Build history of the part. All positions in model axes, mm. Coordinates: 2 decimals unless noted, no trailing zeros. Loops run counter-clockwise (first coordinate to the right, second up) from the corner with the lowest first, then second, coordinate; pieces in that order, holes last.
Item 1: Cut at A-A (x = 63.5). List the corners of the cut face in (y, z) (3 decimals), and give its area (3 significant figures).
Item 2: Mould opens along X. For faces 1 (the face through (48, 12.7, -64)), 2 (the face through (67.315, 14.31, -51.386)), 3 (the face through (45.73, 6.44, -56.52)) say: released by +X, released by -X, zero draft, split by the parting line, or undercut.
Item 3: Cut at C-C (x = 30.5). List the corners of the cut face in (y, z).
Item 4: Drill centre lines: line 1 along Y through (x, z) = (41.5, -44.5); line 2 along X through (y, z) = (10, -51); line 3 along Z through (x, y) = (51.5, 7). Where is each one in solid material? Low to high.
Item 5: Cut at D-D (z = -96.5). List the corners of the cut face in (x, y), and give its area (3 significant figures).
Item 6: Flat gauge pins, fed straight in: pin 1 (3 mm diameter, centred on x = 68.73, z = -45.18, fed in from +Y); pin 2 (4 mm diameter, centred on x = 58.27, z = -45.18, fed in from +Y). Where does each tip first touch, or does it go through?
Item 7: Cut at B-B (z = -63.5). List the corners of the cut face in (x, y) (3 decimals).
from build123d import *

# Parameters (mm, degrees)
SKETCH3_W           = 127
SKETCH3_H           = 127
BOSS_EXTRUDE1_DEPTH = 15.875
SKETCH4_W           = 127
SKETCH4_H           = 127
SKETCH4_R           = 12.7
CUT_EXTRUDE1_DEPTH  = 3.175
CUT_EXTRUDE2_REACH  = 182.054
SKETCH5_R           = 1.8288
CUT_EXTRUDE3_REACH  = 182.054
SKETCH9_R           = 1.8288
CUT_EXTRUDE4_REACH  = 182.054
SKETCH10_R          = 1.8288


with BuildPart() as part:
    # Sketch3 → Boss-Extrude1 (new body)
    with BuildSketch(Plane(origin=(0, 0, 0), x_dir=(1, 0, 0), z_dir=(0, 1, 0))):
        with Locations((63.5, 63.5)):
            Rectangle(SKETCH3_W, SKETCH3_H)
    extrude(amount=BOSS_EXTRUDE1_DEPTH)

    # Sketch4 → Cut-Extrude1 (cut)
    with BuildSketch(Plane(origin=(0, 15.875, 0), x_dir=(1, 0, 0), z_dir=(0, 1, 0))):
        with Locations((63.5, 63.5)):
            Rectangle(SKETCH4_W, SKETCH4_H)
        with Locations(Location((63.5, 63.5, 0), (0, 0, 270))):
            Circle(SKETCH4_R, mode=Mode.SUBTRACT)
    extrude(amount=-CUT_EXTRUDE1_DEPTH, mode=Mode.SUBTRACT)

    # Sketch5 → Cut-Extrude2 (cut, up to next)
    with BuildSketch(Plane(origin=(0, 12.7, 0), x_dir=(1, 0, 0), z_dir=(0, 1, 0)), mode=Mode.PRIVATE) as cut_extrude2_sk1:
        with Locations(Location((45.182968797, 58.266562514, 0), (0, 0, 270))):
            Circle(SKETCH5_R)
    cut_extrude2_tool1 = extrude(cut_extrude2_sk1.sketch, amount=-CUT_EXTRUDE2_REACH, mode=Mode.PRIVATE) & part.part
    # Sketch5 → Cut-Extrude2 (cut, up to next)
    with BuildSketch(Plane(origin=(0, 12.7, 0), x_dir=(1, 0, 0), z_dir=(0, 1, 0)), mode=Mode.PRIVATE) as cut_extrude2_sk2:
        with Locations(Location((68.733437486, 45.182968797, 0), (0, 0, 270))):
            Circle(SKETCH5_R)
    cut_extrude2_tool2 = extrude(cut_extrude2_sk2.sketch, amount=-CUT_EXTRUDE2_REACH, mode=Mode.PRIVATE) & part.part
    # Sketch5 → Cut-Extrude2 (cut, up to next)
    with BuildSketch(Plane(origin=(0, 12.7, 0), x_dir=(1, 0, 0), z_dir=(0, 1, 0)), mode=Mode.PRIVATE) as cut_extrude2_sk3:
        with Locations(Location((81.817031203, 68.733437486, 0), (0, 0, 270))):
            Circle(SKETCH5_R)
    cut_extrude2_tool3 = extrude(cut_extrude2_sk3.sketch, amount=-CUT_EXTRUDE2_REACH, mode=Mode.PRIVATE) & part.part
    # Sketch5 → Cut-Extrude2 (cut, up to next)
    with BuildSketch(Plane(origin=(0, 12.7, 0), x_dir=(1, 0, 0), z_dir=(0, 1, 0)), mode=Mode.PRIVATE) as cut_extrude2_sk4:
        with Locations(Location((58.266562514, 81.817031203, 0), (0, 0, 270))):
            Circle(SKETCH5_R)
    cut_extrude2_tool4 = extrude(cut_extrude2_sk4.sketch, amount=-CUT_EXTRUDE2_REACH, mode=Mode.PRIVATE) & part.part
    add(cut_extrude2_tool1.solids().sort_by_distance((45.182969, 12.7, -58.266563))[0], mode=Mode.SUBTRACT)
    add(cut_extrude2_tool2.solids().sort_by_distance((68.733437, 12.7, -45.182969))[0], mode=Mode.SUBTRACT)
    add(cut_extrude2_tool3.solids().sort_by_distance((81.817031, 12.7, -68.733437))[0], mode=Mode.SUBTRACT)
    add(cut_extrude2_tool4.solids().sort_by_distance((58.266563, 12.7, -81.817031))[0], mode=Mode.SUBTRACT)

    # Sketch9 → Cut-Extrude3 (cut, up to next)
    with BuildSketch(Plane(origin=(0, 12.7, 0), x_dir=(1, 0, 0), z_dir=(0, 1, 0)), mode=Mode.PRIVATE) as cut_extrude3_sk1:
        with Locations(Location((68.733437486, 81.817031203, 0), (0, 0, 270))):
            Circle(SKETCH9_R)
    cut_extrude3_tool1 = extrude(cut_extrude3_sk1.sketch, amount=-CUT_EXTRUDE3_REACH, mode=Mode.PRIVATE) & part.part
    # Sketch9 → Cut-Extrude3 (cut, up to next)
    with BuildSketch(Plane(origin=(0, 12.7, 0), x_dir=(1, 0, 0), z_dir=(0, 1, 0)), mode=Mode.PRIVATE) as cut_extrude3_sk2:
        with Locations(Location((58.266562514, 45.182968797, 0), (0, 0, 270))):
            Circle(SKETCH9_R)
    cut_extrude3_tool2 = extrude(cut_extrude3_sk2.sketch, amount=-CUT_EXTRUDE3_REACH, mode=Mode.PRIVATE) & part.part
    add(cut_extrude3_tool1.solids().sort_by_distance((68.733437, 12.7, -81.817031))[0], mode=Mode.SUBTRACT)
    add(cut_extrude3_tool2.solids().sort_by_distance((58.266563, 12.7, -45.182969))[0], mode=Mode.SUBTRACT)

    # Sketch10 → Cut-Extrude4 (cut, up to next)
    with BuildSketch(Plane(origin=(0, 12.7, 0), x_dir=(1, 0, 0), z_dir=(0, 1, 0)), mode=Mode.PRIVATE) as cut_extrude4_sk1:
        with Locations(Location((76.970384182, 76.970384182, 0), (0, 0, 270))):
            Circle(SKETCH10_R)
    cut_extrude4_tool1 = extrude(cut_extrude4_sk1.sketch, amount=-CUT_EXTRUDE4_REACH, mode=Mode.PRIVATE) & part.part
    # Sketch10 → Cut-Extrude4 (cut, up to next)
    with BuildSketch(Plane(origin=(0, 12.7, 0), x_dir=(1, 0, 0), z_dir=(0, 1, 0)), mode=Mode.PRIVATE) as cut_extrude4_sk2:
        with Locations(Location((50.029615818, 50.029615818, 0), (0, 0, 270))):
            Circle(SKETCH10_R)
    cut_extrude4_tool2 = extrude(cut_extrude4_sk2.sketch, amount=-CUT_EXTRUDE4_REACH, mode=Mode.PRIVATE) & part.part
    add(cut_extrude4_tool1.solids().sort_by_distance((76.970384, 12.7, -76.970384))[0], mode=Mode.SUBTRACT)
    add(cut_extrude4_tool2.solids().sort_by_distance((50.029616, 12.7, -50.029616))[0], mode=Mode.SUBTRACT)


solid = part.part
Filled sheet:
1. outline: (0, -127) - (12.7, -127) - (12.7, -76.2) - (15.875, -76.2) - (15.875, -50.8) - (12.7, -50.8) - (12.7, 0) - (0, 0) - close
1. area: 1,690 mm2
2. face 1: zero draft
2. face 2: split by the parting line
2. face 3: undercut
3. outline: (0, -127) - (12.7, -127) - (12.7, 0) - (0, 0) - close
4. line 1: y = 0 to 12.7
4. line 2: x = 0 to 48.48, 51.58 to 127
4. line 3: z = -127 to -51.12, -48.94 to 0
5. outline: (0, 0) - (127, 0) - (127, 12.7) - (0, 12.7) - close
5. area: 1,610 mm2
6. pin 1: passes through
6. pin 2: stops at y = 12.7
7. outline: (0, 0) - (127, 0) - (127, 12.7) - (76.2, 12.7) - (76.2, 15.875) - (50.8, 15.875) - (50.8, 12.7) - (0, 12.7) - close
